Job drawing, mm, ordinate dimensions from the low corner. One solid piece. A direction names the side the tool comes from. Give positions to 0.01 mm unless a question says otherwise; leave off trailing zeros. Write each loop counter-clockwise with the first axis right and the second up, starting at its lowest first coordinate (ties: lowest second). Pieces come first, ordered by that corner, then holes. Notation, with made-up numbers: (64, 23) - (82, 23) arc R21 ccw to (82, 31) - close; hole circle Ø6 at (11, 14). An arc over 180 degrees is marked (long way). Answer as a JSON object with one key per item and string values.
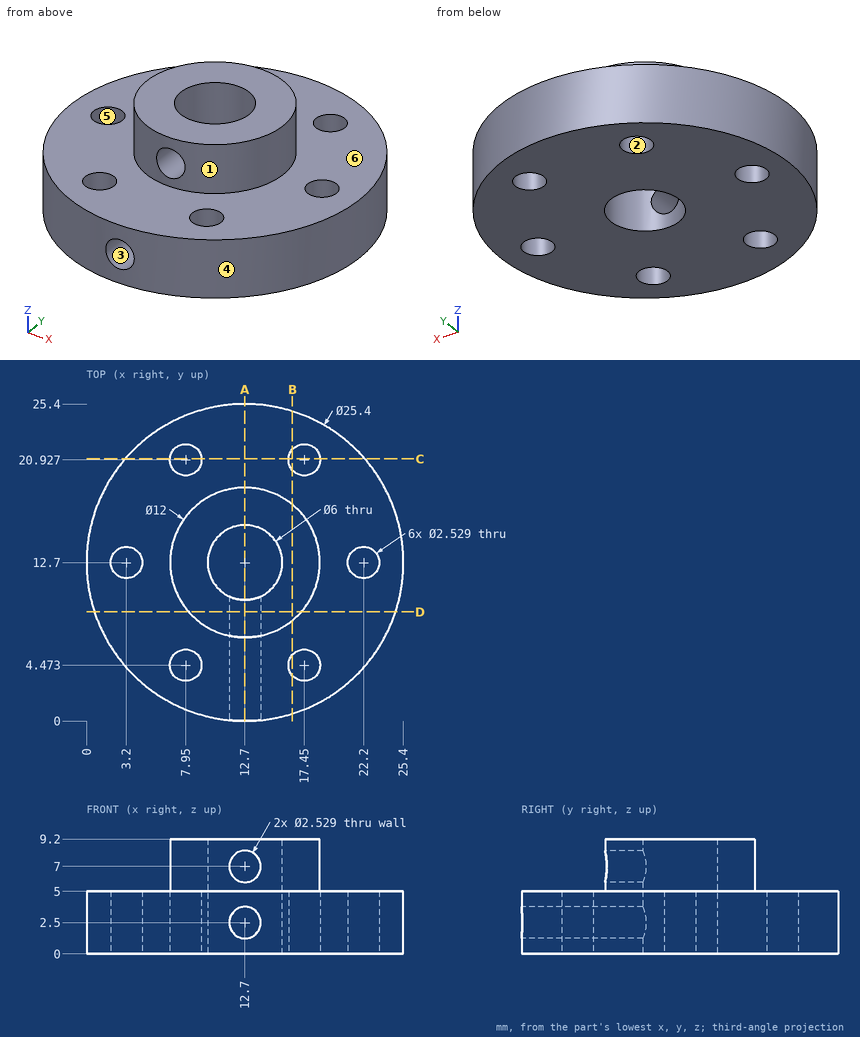
Item 1: Cut at D-D (y = 8.75). Give the cut face in (x, z).
Entries:
{"outline": "(0.63, 0) - (24.77, 0) - (24.77, 5) - (17.22, 5) - (17.22, 9.2) - (8.18, 9.2) - (8.18, 5) - (0.63, 5) - close; hole circle Ø2.53 at (12.7, 2.5); hole circle Ø2.53 at (12.7, 7)"}
Item 2: Probe line 1 (Y direction, x = 12.5, z = 4); line 2 (Y direction, x = 7, z = 3.5); line 3 (Y direction, x = 17.5, z = 4.75). List the from-to ranges inside material, lowest first. Write a range as from..to.
Entries:
{"line 1": "0..9.71, 15.69..25.4", "line 2": "1.35..3.64, 5.31..20.09, 21.76..24.05", "line 3": "0.94..3.21, 5.74..19.66, 22.19..24.46"}
Item 3: Mould opens along X. For the marked faces 4, 5 and 6 say: +X half, -X half, draft (parallel to the pull), parting line (faces both ways), or undercut.
Entries:
{"face 4": "parting line", "face 5": "undercut", "face 6": "draft"}
Item 4: Which spindle directions (+Z, -Z, +X, -X, +Y, -Y) get a long thin tool onto all of the face, cutting with end or side? Do the marked faces 1, 2 and 3. Say none if no direction does.
Entries:
{"face 1": "+Z", "face 2": "+Z, -Z", "face 3": "-Y"}
Item 5: Flat gauge pins, fed straight in: P1, Ø2, axis at x = 19, z = 5, coming from the -Y side; P2, Ø1, axis at x = 3.5, y = 3.5, coming from the +Z side; P3, Ø3, axis at y = 14.5, z = 3.5, coming from the +X side. Where does each tip first touch, or does it go through?
Entries:
{"P1": "y = 1.16", "P2": "z = 5", "P3": "x = 25.4"}
Item 6: Cut at A-A (x = 12.7). Give the cut face in (y, z).
Entries:
{"outline": "(0, 0) - (9.7, 0) - (9.7, 1.24) - (0, 1.24) - close; (0, 3.76) - (9.7, 3.76) - (9.7, 5.74) - (6.7, 5.74) - (6.7, 5) - (0, 5) - close; (6.7, 8.26) - (9.7, 8.26) - (9.7, 9.2) - (6.7, 9.2) - close; (15.7, 0) - (25.4, 0) - (25.4, 5) - (18.7, 5) - (18.7, 9.2) - (15.7, 9.2) - close"}
Item 7: Cut at B-B (x = 16.5). Give the cut face in (y, z), and give its area (4 significant figures).
Entries:
{"outline": "(0.58, 0) - (3.64, 0) - (3.64, 5) - (0.58, 5) - close; (5.31, 0) - (20.09, 0) - (20.09, 5) - (17.34, 5) - (17.34, 9.2) - (8.06, 9.2) - (8.06, 5) - (5.31, 5) - close; (21.76, 0) - (24.82, 0) - (24.82, 5) - (21.76, 5) - close", "area": "143.5 mm2"}
Item 8: Cut at C-C (y = 21). Give the cut face in (x, z).
Entries:
{"outline": "(3.09, 0) - (6.69, 0) - (6.69, 5) - (3.09, 5) - close; (9.21, 0) - (16.19, 0) - (16.19, 5) - (9.21, 5) - close; (18.71, 0) - (22.31, 0) - (22.31, 5) - (18.71, 5) - close"}
